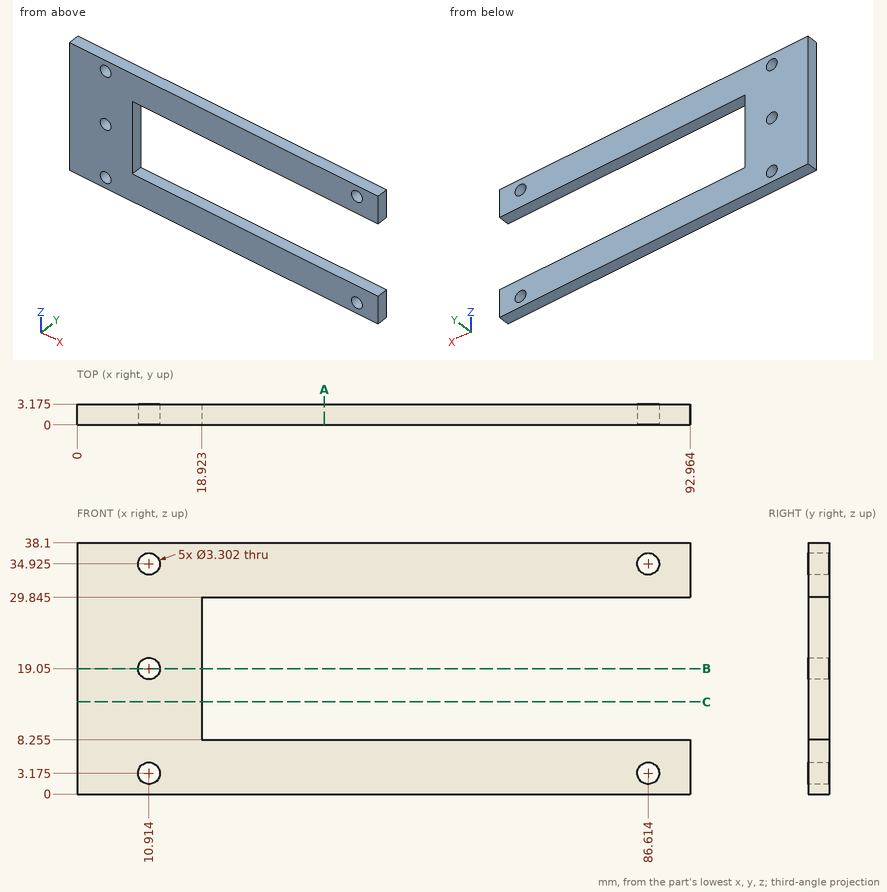
Print and shaded views of the part. All mm, measured from the part's lowest x, y and z. Give positions to 0.01 mm unless a question says otherwise; leave off trailing zeros. Write each loop counter-clockwise with the first axis right and the second up, starting at its lowest first coordinate (ties: lowest second). Pieces come first, ordered by that corner, then holes. Notation, with made-up numbers: M 48,82.5 L 57,82.5 A31 cw 57,110.5 Z; hole C 10,11.5 d3. An arc over 180 degrees is marked long. Use a Markdown table: item, result.
1) Drill centre lines: line 1 (Z direction, x = 56, y = 0.35) (1 decimal); line 2 (Z direction, x = 87, y = 3.05) (1 decimal); line 3 (X direction, y = 2.9, z = 19) (1 decimal). Where is each one in solid material? Low to high. Write a range as from..to.
Responses:
| item | result |
|---|---|
| line 1 | z = 0..8.3, 29.8..38.1 |
| line 2 | z = 0..1.6, 4.8..8.3, 29.8..33.3, 36.5..38.1 |
| line 3 | x = 0..9.3, 12.6..18.9 |
2) Cut at B-B (z = 19.05). List the corners of the cut face in (x, y) (1 decimal).
Responses:
| item | result |
|---|---|
| outline | M 0,0 L 9.3,0 L 9.3,3.2 L 0,3.2 Z; M 12.6,0 L 18.9,0 L 18.9,3.2 L 12.6,3.2 Z |
3) Pin check, flat tips, straight feed: pin 1 (2.5 mm diameter, centred on x = 86.614, z = 3.175, fed in from -Y); pin 2 (1.6 mm diameter, centred on y = 2.5, z = 22, fed in from +X). Stop position of each tip, or through.
Responses:
| item | result |
|---|---|
| pin 1 | passes through |
| pin 2 | stops at x = 18.92 |
4) Cut at A-A (x = 37.5). List the corners of the cut face in (y, z) (1 decimal), and give its area (3 significant figures).
Responses:
| item | result |
|---|---|
| outline | M 0,0 L 3.2,0 L 3.2,8.3 L 0,8.3 Z; M 0,29.8 L 3.2,29.8 L 3.2,38.1 L 0,38.1 Z |
| area | 52.4 mm2 |
5) Cut at C-C (z = 14). List the corners of the cut face in (x, y) (1 decimal), and give its area (3 significant figures).
Responses:
| item | result |
|---|---|
| outline | M 0,0 L 18.9,0 L 18.9,3.2 L 0,3.2 Z |
| area | 60.1 mm2 |
